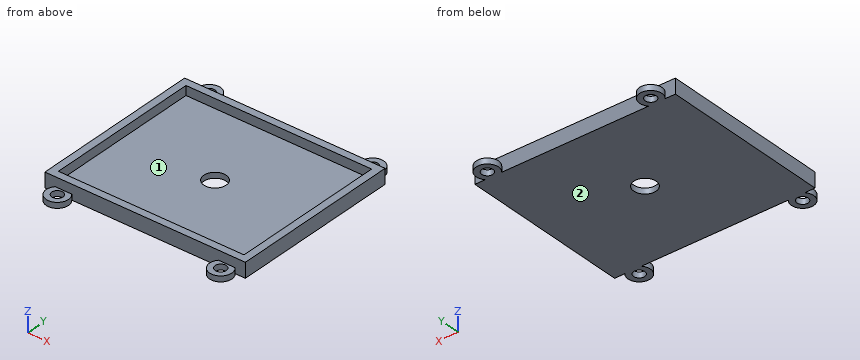
```python
from build123d import *

# Parameters (mm, degrees)
SKETCH_W         = 54
SKETCH_H         = 46
SKETCH_W_2       = 50
SKETCH_H_2       = 42
EXTRUDE001_DEPTH = 4
SKETCH001_R      = 1.5
SKETCH001_R_2    = 3
EXTRUDE_DEPTH    = 1.5


with BuildPart() as extrude001:
    # Sketch → Extrude001 (new body)
    with BuildSketch(Plane.XY.offset(1.5)):
        Rectangle(SKETCH_W, SKETCH_H)
        Rectangle(SKETCH_W_2, SKETCH_H_2, mode=Mode.SUBTRACT)
    extrude(amount=EXTRUDE001_DEPTH)


with BuildPart() as fusion:
    # Sketch001 (on Sketch) → Extrude (new body)
    with BuildSketch(Plane.XY.offset(1.5)):
        with BuildLine():
            Line((27, 23), (27, -23))
            Line((27, -23), (24.236068, -23))
            ThreePointArc((19.763932, -23), (22, -28), (24.236068, -23))
            Line((19.763932, -23), (-19.763932, -23))
            ThreePointArc((-24.236068, -23), (-22, -28), (-19.763932, -23))
            Line((-24.236068, -23), (-27, -23))
            Line((-27, -23), (-27, 23))
            Line((-24.236068, 23), (-27, 23))
            ThreePointArc((-19.763932, 23), (-22, 28), (-24.236068, 23))
            Line((-19.763932, 23), (19.763932, 23))
            ThreePointArc((24.236068, 23), (22, 28), (19.763932, 23))
            Line((24.236068, 23), (27, 23))
        make_face()
        with Locations((-22, 25)):
            Circle(SKETCH001_R, mode=Mode.SUBTRACT)
        with Locations((22, 25)):
            Circle(SKETCH001_R, mode=Mode.SUBTRACT)
        with Locations((-22, -25)):
            Circle(SKETCH001_R, mode=Mode.SUBTRACT)
        with Locations((22, -25)):
            Circle(SKETCH001_R, mode=Mode.SUBTRACT)
        Circle(SKETCH001_R_2, mode=Mode.SUBTRACT)
    extrude(amount=EXTRUDE_DEPTH)

    # Fusion: union Extrude001
    add(extrude001.part)


solid = fusion.part
```
Verification items for the finished model (mm, model axes). Face numbers are marked on the shaded views. Coordinates: 2 decimals unless noted, no trailing zeros. Loops run counter-clockwise (first coordinate to the right, second up) from the corner with the lowest first, then second, coordinate; pieces in that order, holes last. Notation, with made-up numbers: (24, -34.75) -> (38, -34.75) arc R26 ccw to (38, -11.75) -> close; hole circle Ø1 at (85.25, 77). An arc over 180 degrees is marked (long way). Put each result on its own line as item: value.
1. Thickness scan on line 1 (Y direction, x = -22, z = 2); line 2 (Y direction, x = 0, z = 1.9); line 3 (Y direction, x = -19, z = 3.3). Record the ranges inside material, lowest first.
Result set:
line 1: y = -28 to -26.5, -23.5 to 23.5, 26.5 to 28
line 2: y = -23 to -3, 3 to 23
line 3: y = -23 to -21, 21 to 23
2. Section check D-D, the plane x = 0. Record the boundary of the cut face in (y, z), then the cut area to 3 significant figures.
Result set:
outline: (-23, 1.5) -> (-3, 1.5) -> (-3, 3) -> (-21, 3) -> (-21, 5.5) -> (-23, 5.5) -> close; (3, 1.5) -> (23, 1.5) -> (23, 5.5) -> (21, 5.5) -> (21, 3) -> (3, 3) -> close
area: 70.0 mm^2
3. Section check C-C, the plane z = 4.05. Record the boundary of the cut face in (x, y), then the cut area to 3 significant figures.
Result set:
outline: (-27, -23) -> (27, -23) -> (27, 23) -> (-27, 23) -> close; hole (-25, -21) -> (25, -21) -> (25, 21) -> (-25, 21) -> close
area: 384 mm^2
4. Section check A-A, the plane x = 22. Record the boundary of the cut face in (y, z).
Result set:
outline: (-28, 1.5) -> (-26.5, 1.5) -> (-26.5, 3) -> (-28, 3) -> close; (-23.5, 1.5) -> (23.5, 1.5) -> (23.5, 3) -> (23, 3) -> (23, 5.5) -> (21, 5.5) -> (21, 3) -> (-21, 3) -> (-21, 5.5) -> (-23, 5.5) -> (-23, 3) -> (-23.5, 3) -> close; (26.5, 1.5) -> (28, 1.5) -> (28, 3) -> (26.5, 3) -> close
5. Mould release check, pull along Y, two halves, no side actions. Record for the marked faces 1 and 2: pulls with the +Y half, pulls with the -Y half, needs draft (parallel to the pull), parting line crosses it, or undercut.
Result set:
face 1: undercut
face 2: needs draft
6. Section check B-B, the plane y = 0. Record the boundary of the cut face in (x, z).
Result set:
outline: (-27, 1.5) -> (-3, 1.5) -> (-3, 3) -> (-25, 3) -> (-25, 5.5) -> (-27, 5.5) -> close; (3, 1.5) -> (27, 1.5) -> (27, 5.5) -> (25, 5.5) -> (25, 3) -> (3, 3) -> close
7. Gauge pin test, flat ends, axial feed: P1, Ø4, axis at x = -22.5, y = -25.5, coming from the +Z side; P2, Ø2.5, axis at x = -22, y = -25, coming from the -Z side; P3, Ø1, axis at x = 7, z = 2.5, coming from the -Y side; P4, Ø0.8, axis at x = -8.5, z = 4, coming from the +Y side. Record the tip position at first contact, or that the pin passes through.
Result set:
P1: stops at z = 3
P2: passes through
P3: stops at y = -23
P4: stops at y = 23
